Source: CAD feature listing. Evaluate the final solid. Frame: model axes, mm. Give positions to 0.01 mm unless a question says otherwise; leave off trailing zeros. Write each loop counter-clockwise with the first axis right and the second up, starting at its lowest first coordinate (ties: lowest second). Pieces come first, ordered by that corner, then holes. Notation, with made-up numbers: (64, 81) -> (92, 81) arc R14 ccw to (92, 86) -> close; hole circle Ø1 at (57.25, 80). An arc over 180 degrees is marked (long way). Use a Markdown table: item, result. Add a question column.
```python
from build123d import *

# Parameters (mm, degrees)
SKETCH1_R           = 69.85
BOSS_EXTRUDE1_DEPTH = 12.7
SKETCH1_3_R         = 69.85
SKETCH1_3_R_2       = 63.5
BOSS_EXTRUDE2_DEPTH = 227.965
SKETCH2_R           = 69.85
BOSS_EXTRUDE3_DEPTH = 12.7
SKETCH3_R           = 8.9296875
CUT_EXTRUDE1_DEPTH  = 335.534


with BuildPart() as part:
    # Sketch1 → Boss-Extrude1 (new body)
    with BuildSketch(Plane(origin=(0, 0, 0), x_dir=(1, 0, 0), z_dir=(0, 1, 0))):
        with Locations(Location((0, 0, 0), (0, 0, 270))):
            Circle(SKETCH1_R)
    extrude(amount=BOSS_EXTRUDE1_DEPTH)

    # Sketch1_3 → Boss-Extrude2 (add)
    with BuildSketch(Plane(origin=(0, 0, 0), x_dir=(1, 0, 0), z_dir=(0, 1, 0))):
        with Locations(Location((0, 0, 0), (0, 0, 270))):
            Circle(SKETCH1_3_R)
        with Locations(Location((0, 0, 0), (0, 0, 270))):
            Circle(SKETCH1_3_R_2, mode=Mode.SUBTRACT)
    extrude(amount=BOSS_EXTRUDE2_DEPTH)

    # Sketch2 → Boss-Extrude3 (add)
    with BuildSketch(Plane(origin=(0, 227.965, 0), x_dir=(1, 0, 0), z_dir=(0, 1, 0))):
        with Locations(Location((0, 0, 0), (0, 0, 270))):
            Circle(SKETCH2_R)
    extrude(amount=BOSS_EXTRUDE3_DEPTH)

    # Sketch3 → Cut-Extrude1 (cut)
    with BuildSketch(Plane(origin=(0, 240.665, 0), x_dir=(1, 0, 0), z_dir=(0, 1, 0))):
        with Locations(Location((0, 0, 0), (0, 0, 270))):
            Circle(SKETCH3_R)
    extrude(amount=-CUT_EXTRUDE1_DEPTH, mode=Mode.SUBTRACT)


solid = part.part
```
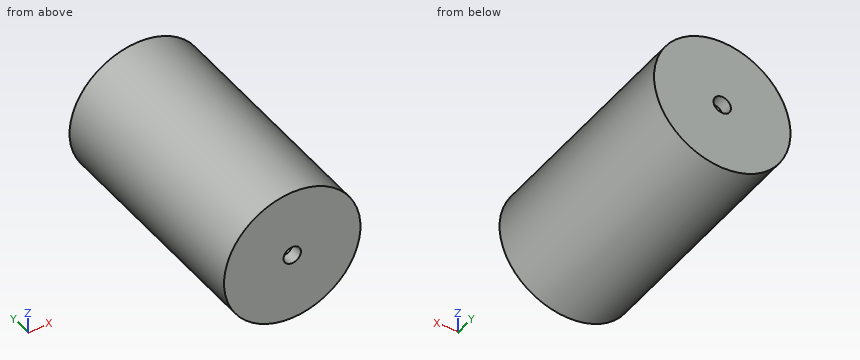
(1) First-contact query: pin 1 Ø1.5 at (x, y) = (26, 73.5) entering from -Z; pin 2 Ø4 at (x, y) = (26.5, 174) entering from -Z; pin 3 Ø8 at (x, y) = (-37, 101.5) entering from -Z. Flat tips, straight axial feed; report the tip coordinate or a pass-through.
(2) Cut plane B-B on x = 0. Return the cut outline in (y, z) (3 decimals).
(3) Cut plane D-D on z = 49.5. Return the cut outline in (x, y) (3 decimals), then the cut area to 3 significant figures.
(4) Material intervals for L1, parallel to X at y = 233.5, z = 0; L2, parallel to Y at x = 58, z = 15.5 (3 decimals); L3, parallel to X at y = 168.5, z = 0, sorted ascending.
(5) Cut plane A-A on z = 0. Return the cut outline in (x, y) (3 decimals), then the cut area to 3 significant figures.
(6) Cut plane C-C on y = 198. Return the cut outline in (x, z).
Output:
| question | item | result |
|---|---|---|
| 1 | pin 1 | z = -65.13 |
| 1 | pin 2 | z = -65.41 |
| 1 | pin 3 | z = -61.56 |
| 2 | outline | (0, -69.85) -> (240.665, -69.85) -> (240.665, -8.93) -> (227.965, -8.93) -> (227.965, -63.5) -> (12.7, -63.5) -> (12.7, -8.93) -> (0, -8.93) -> close; (0, 8.93) -> (12.7, 8.93) -> (12.7, 63.5) -> (227.965, 63.5) -> (227.965, 8.93) -> (240.665, 8.93) -> (240.665, 69.85) -> (0, 69.85) -> close |
| 3 | outline | (-49.283, 0) -> (49.283, 0) -> (49.283, 240.665) -> (-49.283, 240.665) -> close; hole (-39.774, 12.7) -> (39.774, 12.7) -> (39.774, 227.965) -> (-39.774, 227.965) -> close |
| 3 | area | 6,600 mm^2 |
| 4 | L1 | -69.85 to -8.93, 8.93 to 69.85 |
| 4 | L2 | 0 to 12.7, 227.965 to 240.665 |
| 4 | L3 | -69.85 to -63.5, 63.5 to 69.85 |
| 5 | outline | (-69.85, 0) -> (-8.93, 0) -> (-8.93, 12.7) -> (-63.5, 12.7) -> (-63.5, 227.965) -> (-8.93, 227.965) -> (-8.93, 240.665) -> (-69.85, 240.665) -> close; (8.93, 0) -> (69.85, 0) -> (69.85, 240.665) -> (8.93, 240.665) -> (8.93, 227.965) -> (63.5, 227.965) -> (63.5, 12.7) -> (8.93, 12.7) -> close |
| 5 | area | 5,830 mm^2 |
| 6 | outline | circle Ø139.7 at (0, 0); hole circle Ø127 at (0, 0) |
